from build123d import *

# Parameters (mm, degrees)
CROQUIS1_W              = 240
CROQUIS1_H              = 240
SALIENTE_EXTRUIR1_DEPTH = 6.35
CROQUIS2_W              = 88.9
CROQUIS2_H              = 88.9
SALIENTE_EXTRUIR2_DEPTH = 900
CROQUIS3_W              = 550
CROQUIS3_H              = 400
SALIENTE_EXTRUIR3_DEPTH = 320
CORTAR_EXTRUIR1_DEPTH   = 550
CROQUIS6_W              = 355.6
CROQUIS6_H              = 203.2
CORTAR_EXTRUIR2_DEPTH   = 90


with BuildPart() as part:
    # Croquis1 → Saliente-Extruir1 (new body)
    with BuildSketch(Plane(origin=(0, 0, 0), x_dir=(1, 0, 0), z_dir=(0, 1, 0))):
        with Locations((120, 120)):
            Rectangle(CROQUIS1_W, CROQUIS1_H)
    extrude(amount=SALIENTE_EXTRUIR1_DEPTH)

    # Croquis2 → Saliente-Extruir2 (add)
    with BuildSketch(Plane(origin=(0, 6.35, 0), x_dir=(1, 0, 0), z_dir=(0, 1, 0))):
        with Locations((120, 120)):
            Rectangle(CROQUIS2_W, CROQUIS2_H)
    extrude(amount=SALIENTE_EXTRUIR2_DEPTH)

    # Croquis3 → Saliente-Extruir3 (add)
    with BuildSketch(Plane(origin=(0, 906.35, 0), x_dir=(1, 0, 0), z_dir=(0, 1, 0))):
        with Locations((120, 120)):
            Rectangle(CROQUIS3_W, CROQUIS3_H)
    extrude(amount=SALIENTE_EXTRUIR3_DEPTH)

    # Croquis4 → Cortar-Extruir1 (cut)
    with BuildSketch(Plane.ZY.offset(155)):
        Polygon((-320, 1226.35), (80, 996.35), (80, 1226.35), align=None)
    extrude(amount=-CORTAR_EXTRUIR1_DEPTH, mode=Mode.SUBTRACT)

    # Croquis6 → Cortar-Extruir2 (cut)
    with BuildSketch(Plane(origin=(0, 783.353687177, 450.428370127), x_dir=(1, 0, 0), z_dir=(0, 0.8669063030575354, 0.4984711242580827))):
        with Locations((120, 658.004640311)):
            Rectangle(CROQUIS6_W, CROQUIS6_H)
    extrude(amount=-CORTAR_EXTRUIR2_DEPTH, mode=Mode.SUBTRACT)


solid = part.part
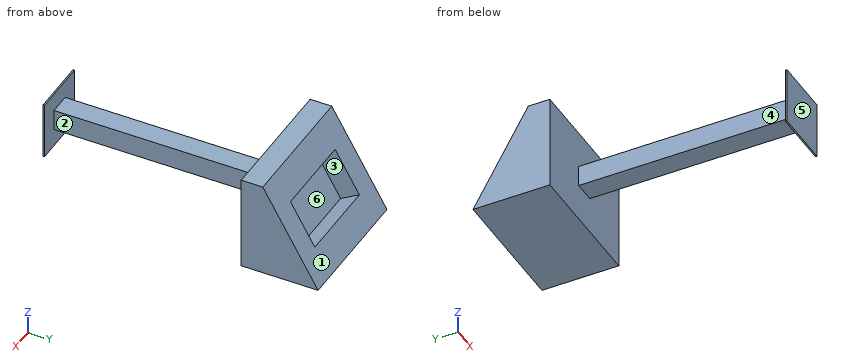
Geometry: final body of the model. Coordinates: model frame, mm. Face numbers are marked on the shaded views. A direction names the side the tool comes from. Round coordinates to 2 decimals unless told otherwise and drop trailing zeros. Order: outer loops, then holes, each group sorted by start corner. A loop starts at its lowest first (then second) coordinate and runs counter-clockwise, first axis right, second up.
Q1. Mould query, pull axis X, two halves, no side actions, for the marked faces 1, 2 and 3. Classes: released by +X, released by -X, zero draft, split by the parting line, or undercut.
Result sheet:
face 1: zero draft
face 2: released by +X
face 3: undercut
Q2. Section B-B, the plane y = 1040. Output: boundary loops of the cut face in (x, z).
Result sheet:
outline: (-155, -320) - (395, -320) - (395, 4.09) - (-155, 4.09) - close; hole (-57.8, -176.47) - (297.8, -176.47) - (297.8, -43.83) - (-57.8, -43.83) - close
Q3. Section C-C, the plane z = -181. Output: boundary loops of the cut face in (x, y) (3 decimals), and give its area (3 significant figures).
Result sheet:
outline: (-155, 906.35) - (395, 906.35) - (395, 1146.425) - (297.8, 1146.425) - (297.8, 1042.608) - (-57.8, 1042.608) - (-57.8, 1146.425) - (-155, 1146.425) - close; (0, 0) - (240, 0) - (240, 6.35) - (0, 6.35) - close
area: 96,600 mm2
Q4. Section D-D, the plane x = 270. Output: boundary loops of the cut face in (y, z).
Result sheet:
outline: (906.35, -320) - (1226.35, -320) - (1161.99, -208.08) - (1083.97, -252.94) - (982.68, -76.78) - (1060.71, -31.92) - (996.35, 80) - (906.35, 80) - close
Q5. Pin query (flat end, axial travel): pin 1 (10 mm diameter, centred on y = 616.5, z = -119.5, fed in from +X); pin 2 (5 mm diameter, centred on x = 88, y = 2, fed in from -Z); pin 3 (7 mm diameter, centred on y = 3.5, z = -160.5, fed in from -X). Return the tip coordinate at first contact, or that it passes through.
Result sheet:
pin 1: stops at x = 164.45
pin 2: stops at z = -240
pin 3: stops at x = 0
Q6. Access query for the marked faces 4, 5 and 6. Directions: +Z, -Z, +X, -X, +Y, -Y. A direction counts if a zero-diameter tool reaches every point of the face in a straight line with its end or side. Return the directions, or none.
Result sheet:
face 4: +Z, -Z, -X
face 5: +Z, -Z, +X, -X, -Y
face 6: none
Q7. Material intervals for probe 1 along X at (y, z) = (1141.5, -201); probe 2 along X at (y, z) = (790.5, -161); probe 3 along Y at (x, z) = (2, -146), sorted ascending.
Result sheet:
probe 1: x = -155 to -57.8, 297.8 to 395
probe 2: x = 75.55 to 164.45
probe 3: y = 0 to 6.35, 906.35 to 1022.48
Q8. Section A-A, the plane x = 54. Output: boundary loops of the cut face in (y, z).
Result sheet:
outline: (0, -240) - (6.35, -240) - (6.35, 0) - (0, 0) - close; (906.35, -320) - (1226.35, -320) - (1161.99, -208.08) - (1083.97, -252.94) - (982.68, -76.78) - (1060.71, -31.92) - (996.35, 80) - (906.35, 80) - close
